Autodesk Fusion 360 part; units mm, degrees
sketch "Sketch1" plane through (0, 0, 0) normal (0, 0, 1) x (1, 0, 0)
  line L0 (0, 0) -> (53.9524, 0)
  line L1 (53.9524, 0) -> (53.9524, 14.5545)
  line L2 (35.7878, 32.7191) -> (0, 32.7191)
  line L3 (0, 32.7191) -> (0, 0)
  arc A0 (35.7878, 32.7191) -> (53.9524, 14.5545) centre (53.9524, 32.7191) ccw
extrude "Extrude1" add sketch "Sketch1" along normal blind 18.598
sketch "Sketch2" plane through (0, 0, 18.598) normal (0, 0, 1) x (-1, 0, 0)
  line L0 (0, 0) -> (-18.618, 0)
  line L1 (-18.618, 0) -> (-18.618, -15.1183)
  line L2 (-18.618, -15.1183) -> (0, -15.1183)
  line L3 (0, -15.1183) -> (0, 0)
extrude "Extrude2" add sketch "Sketch2" along normal blind 15.729
fillet "Fillet1" radius 9.525 1 edges at (18.618, 15.1183, 26.4625)
fillet "Fillet2" radius 8.158 1 edges at (0, 0, 17.1635)
ref_plane "WorkPlane1" through (0, 0, 45.086) normal (0, 0, 1) x (1, 0, 0)
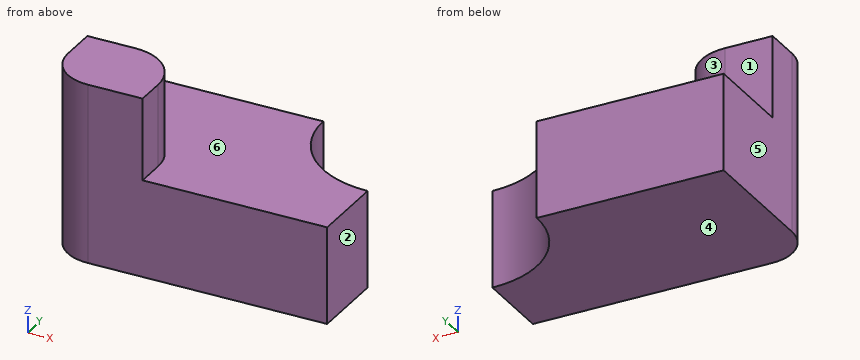
Input: part model. Units: mm. Frame: model coordinates. Face numbers are marked on the shaded views. A direction names the side the tool comes from. Coordinates: 2 decimals unless noted, no trailing zeros. Loops run counter-clockwise (first coordinate to the right, second up) from the corner with the lowest first, then second, coordinate; pieces in that order, holes last.
Q1. Cut plane C-C (y = 5). Output: boundary loops of the cut face in (x, z).
Q2. Material intervals for line 1 (Z direction, x = 42.5, y = 17); line 2 (Y direction, x = 8.5, z = 24.5); line 3 (X direction, y = 21, z = 5), sorted ascending.
Q3. Cut plane A-A (z = 23). Output: boundary loops of the cut face in (x, y) (3 decimals).
Q4. Draft query along Z for the marked faces 4, 5 and 6. Return one class per face: +Z half, -Z half, draft (parallel to the pull), parting line (faces both ways), or undercut.
Q5. Cut plane B-B (x = 30). Output: boundary loops of the cut face in (y, z), then the cut area to 3 significant figures.
Q6. Set-up query: the marked faces 1, 2 and 3. Return all of +Z, -Z, +X, -X, +Y, -Y with unobstructed straight access to the full face (end or side cutting, diameter ignored); none if empty.
Q7. Contact query for flat-ended pins moving along their axis: pin 1 (1.5 mm diameter, centred on x = 35.5, z = 19, fed in from -Y); pin 2 (6 mm diameter, centred on x = 41.5, y = 20, fed in from +Z); pin 3 (1.7 mm diameter, centred on y = 1.5, z = 30, fed in from +X); pin 4 (4.5 mm diameter, centred on x = 2.5, z = 27, fed in from +Y). Output: stop coordinate, or through.
Q8. Cut plane D-D (x = 48.5). Output: boundary loops of the cut face in (y, z), then the cut area to 3 significant figures.
Working result:
1. outline: (0.64, 0) - (53.95, 0) - (53.95, 18.6) - (18.62, 18.6) - (18.62, 34.33) - (0.64, 34.33) - close
2. line 1: z = 0 to 18.6
2. line 2: y = 0 to 15.12
2. line 3: x = 0 to 40.07
3. outline: (0, 8.158) arc R8.158 ccw to (8.158, 0) - (18.618, 0) - (18.618, 5.593) arc R9.525 ccw to (9.093, 15.118) - (0, 15.118) - close
4. face 4: -Z half
4. face 5: draft
4. face 6: +Z half
5. outline: (0, 0) - (32.72, 0) - (32.72, 18.6) - (0, 18.6) - close
5. area: 609 mm2
6. face 1: +Z, +X, -X, +Y
6. face 2: +Z, -Z, +X, +Y, -Y
6. face 3: +Z, +X, +Y
7. pin 1: stops at y = 0
7. pin 2: stops at z = 18.6
7. pin 3: stops at x = 18.62
7. pin 4: stops at y = 15.12
8. outline: (0, 0) - (15.39, 0) - (15.39, 18.6) - (0, 18.6) - close
8. area: 286 mm2
